Autodesk Inventor part; units mm, degrees
ref_plane "Integral_Raised_Device_Mounting_Boss_StartPlane" through (0, 0, 4) normal (0, 0, 1) x (1, 0, 0)
ref_plane "Device_Clamp_Face_PositiveX" through (33.2942, 0, 0) normal (1, 0, 0) x (0, 1, 0)
ref_plane "Device_Clamp_Face_NegativeX" through (19.7942, 0, 0) normal (1, 0, 0) x (0, 1, 0)
sketch "Continuous_Solid_Plate_No_Openings_Profile" plane through (0, 0, 0) normal (0, 0, 1) x (1, 0, 0)
  line L0 (0, 0) -> (51, 0)
  line L1 (51, 0) -> (51, 80)
  line L2 (51, 80) -> (0, 80)
  line L3 (0, 80) -> (0, 0)
  dimension "d0" = 51
  dimension "d1" = 80
extrude "Continuous_Solid_Plate_No_Openings" add sketch "Continuous_Solid_Plate_No_Openings_Profile" along normal blind 4
ref_plane "Integral_Raised_Device_Mounting_Boss_StartPlane" through (0, 0, 4) normal (0, 0, 1) x (1, 0, 0)
sketch "Integral_Raised_Device_Mounting_Boss_Profile" plane through (0, 0, 4) normal (0, 0, 1) x (1, 0, 0)
  line L0 (19.7942, 4) -> (33.2942, 4)
  line L1 (33.2942, 4) -> (33.2942, 76)
  line L2 (33.2942, 76) -> (19.7942, 76)
  line L3 (19.7942, 76) -> (19.7942, 4)
  point P0 (0, 0)
  dimension "d5" = 19.7943
  dimension "d6" = 4
  dimension "d7" = 13.5
  dimension "d8" = 72
extrude "Integral_Raised_Device_Mounting_Boss" add sketch "Integral_Raised_Device_Mounting_Boss_Profile" along normal blind 6
sketch "Rod_M3_Clearance_8x_Locations" plane through (0, 0, 0) normal (0, 0, 1) x (1, 0, 0)
  circle A0 centre (3, 5) radius 1.7
  circle A1 centre (3, 25) radius 1.7
  circle A2 centre (3, 45) radius 1.7
  circle A3 centre (3, 65) radius 1.7
  circle A4 centre (48, 5) radius 1.7
  circle A5 centre (48, 25) radius 1.7
  circle A6 centre (48, 45) radius 1.7
  circle A7 centre (48, 65) radius 1.7
  point P0 (0, 0)
  dimension "d11" = 3
  dimension "d12" = 5
  dimension "d13" = 3.4
  dimension "d14" = 3
  dimension "d15" = 25
  dimension "d16" = 3.4
  dimension "d17" = 3
  dimension "d18" = 45
  dimension "d19" = 3.4
  dimension "d20" = 3
  dimension "d21" = 65
  dimension "d22" = 3.4
  dimension "d23" = 48
  dimension "d24" = 5
  dimension "d25" = 3.4
  dimension "d26" = 48
  dimension "d27" = 25
  dimension "d28" = 3.4
  dimension "d29" = 48
  dimension "d30" = 45
  dimension "d31" = 3.4
  dimension "d32" = 48
  dimension "d33" = 65
  dimension "d34" = 3.4
extrude "Rod_M3_Clearance_8x" cut sketch "Rod_M3_Clearance_8x_Locations" along normal through all
ref_plane "Device_Clamp_Face_PositiveX" through (33.2942, 0, 0) normal (1, 0, 0) x (0, 1, 0)
sketch "M3_Side_Tap_Locations_PositiveX" plane through (33.2942, 0, 0) normal (1, 0, 0) x (0, 1, 0)
  circle A0 centre (9.828, 7) radius 1.25
  circle A1 centre (25.828, 7) radius 1.25
  circle A2 centre (41.828, 7) radius 1.25
  circle A3 centre (57.828, 7) radius 1.25
  circle A4 centre (73.828, 7) radius 1.25
  point P0 (0, 0)
  dimension "d38" = 9.828
  dimension "d39" = 7
  dimension "d40" = 2.5
  dimension "d41" = 25.828
  dimension "d42" = 7
  dimension "d43" = 2.5
  dimension "d44" = 41.828
  dimension "d45" = 7
  dimension "d46" = 2.5
  dimension "d47" = 57.828
  dimension "d48" = 7
  dimension "d49" = 2.5
  dimension "d50" = 73.828
  dimension "d51" = 7
  dimension "d52" = 2.5
extrude "Device_Tap_Drills_5x_PositiveX" cut sketch "M3_Side_Tap_Locations_PositiveX" against normal blind 6
thread "Device_M3x0_5_6H_PositiveX_1"
thread "Device_M3x0_5_6H_PositiveX_2"
thread "Device_M3x0_5_6H_PositiveX_3"
thread "Device_M3x0_5_6H_PositiveX_4"
thread "Device_M3x0_5_6H_PositiveX_5"
ref_plane "Device_Clamp_Face_NegativeX" through (19.7942, 0, 0) normal (1, 0, 0) x (0, 1, 0)
sketch "M3_Side_Tap_Locations_NegativeX" plane through (19.7942, 0, 0) normal (1, 0, 0) x (0, 1, 0)
  circle A0 centre (9.828, 7) radius 1.25
  circle A1 centre (25.828, 7) radius 1.25
  circle A2 centre (41.828, 7) radius 1.25
  circle A3 centre (57.828, 7) radius 1.25
  circle A4 centre (73.828, 7) radius 1.25
  point P0 (0, 0)
  dimension "d66" = 9.828
  dimension "d67" = 7
  dimension "d68" = 2.5
  dimension "d69" = 25.828
  dimension "d70" = 7
  dimension "d71" = 2.5
  dimension "d72" = 41.828
  dimension "d73" = 7
  dimension "d74" = 2.5
  dimension "d75" = 57.828
  dimension "d76" = 7
  dimension "d77" = 2.5
  dimension "d78" = 73.828
  dimension "d79" = 7
  dimension "d80" = 2.5
extrude "Device_Tap_Drills_5x_NegativeX" cut sketch "M3_Side_Tap_Locations_NegativeX" along normal blind 6
thread "Device_M3x0_5_6H_NegativeX_1"
thread "Device_M3x0_5_6H_NegativeX_2"
thread "Device_M3x0_5_6H_NegativeX_3"
thread "Device_M3x0_5_6H_NegativeX_4"
thread "Device_M3x0_5_6H_NegativeX_5"
equation "\"d0\" = OverallWidth"
equation "\"d1\" = ContactLength"
equation "\"d2\" = BaseThickness"
equation "\"d7\" = FingerWidth"
equation "\"d8\" = ContactLength - 2 * FingerEndInset"
equation "\"d9\" = FingerThickness"
equation "\"d13\" = RodClearanceDiameter"
equation "\"d16\" = RodClearanceDiameter"
equation "\"d19\" = RodClearanceDiameter"
equation "\"d22\" = RodClearanceDiameter"
equation "\"d25\" = RodClearanceDiameter"
equation "\"d28\" = RodClearanceDiameter"
equation "\"d31\" = RodClearanceDiameter"
equation "\"d34\" = RodClearanceDiameter"
equation "\"d40\" = TapDrillDiameter"
equation "\"d43\" = TapDrillDiameter"
equation "\"d46\" = TapDrillDiameter"
equation "\"d49\" = TapDrillDiameter"
equation "\"d52\" = TapDrillDiameter"
equation "\"d53\" = TapDepth"
equation "\"d55\" = TapDepth"
equation "\"d57\" = TapDepth"
equation "\"d59\" = TapDepth"
equation "\"d61\" = TapDepth"
equation "\"d63\" = TapDepth"
equation "\"d68\" = TapDrillDiameter"
equation "\"d71\" = TapDrillDiameter"
equation "\"d74\" = TapDrillDiameter"
equation "\"d77\" = TapDrillDiameter"
equation "\"d80\" = TapDrillDiameter"
equation "\"d81\" = TapDepth"
equation "\"d83\" = TapDepth"
equation "\"d85\" = TapDepth"
equation "\"d87\" = TapDepth"
equation "\"d89\" = TapDepth"
equation "\"d91\" = TapDepth"
equation "\"OverallWidth\" = 51"
equation "\"RodWidth\" = 6"
equation "\"ContactLength\" = 80"
equation "\"BaseThickness\" = 4"
equation "\"FingerStartX\" = 19.79425"
equation "\"FingerWidth\" = 13.5"
equation "\"FingerThickness\" = 6"
equation "\"FingerEndInset\" = 4"
equation "\"RodClearanceDiameter\" = 3.4"
equation "\"ClampFirstY\" = 41.82802"
equation "\"ClampPitch\" = 16"
equation "\"ClampHeight\" = 7"
equation "\"TapDrillDiameter\" = 2.5"
equation "\"TapDepth\" = 6"
equation "\"RodHoleStart\" = 5"
equation "\"RodScrewPitch\" = 20"
equation "\"d4\" = BaseThickness"
equation "\"d37\" = FingerStartX + FingerWidth"
equation "\"d65\" = FingerStartX"
properties part number "Rod_Holder_Adapter"
Check sheet for the modelled part. Datum: model origin and axes. Units: mm. A direction names the side the tool comes from. Round coordinates to 2 decimals unless told otherwise and drop trailing zeros. Order: outer loops, then holes, each group sorted by start corner. A loop starts at its lowest first (then second) coordinate and runs counter-clockwise, first axis right, second up. Notation, with made-up numbers: (-0.5, -14.75) - (27.5, -14.75) arc R31 ccw to (27.5, 19.25) - close; hole circle Ø8 at (70.5, 18). An arc over 180 degrees is marked (long way). Answer as CSV lines item,"result". Start each with the question number.
1) Tool access check on faces 1 (the face through (25.794, 10, 7)), 2 (the face through (51, 39, 2)), 3 (the face through (27.294, 10, 7)). Record the directions out of +Z, -Z, +X, -X, +Y, -Y that give a thin tool (end or side, any length) a straight path to the whole face; none if there is none.
2) Section check D-D (x = 3). Record the cut outline in (y, z), then the cut area to 3 significant figures.
3) Scan lines: probe 1 along Y at (x, z) = (3, 3); probe 2 along X at (y, z) = (45, 2.6); probe 3 along Z at (x, y) = (9, 7). Record each from-to range of solid material in increasing order.
4) Draft check along Z on faces 4 (the face through (22.752, 74.983, 7.479)), 5 (the face through (22.752, 8.836, 7.761)), 6 (the face through (46.75, 63.85, 1.97)). Enter one of: +Z half, -Z half, draft (parallel to the pull), parting line (faces both ways), or undercut.
5) Section check A-A (y = 45). Record the cut outline in (x, z), then the cut area to 3 significant figures.
6) Depth check by flat-ended pin: pin 1 (1.5 mm diameter, centred on y = 57.828, z = 7, fed in from +X); pin 2 (4 mm diameter, centred on x = 48, y = 65, fed in from +Z); pin 3 (4 mm diameter, centred on x = 18, y = 20, fed in from -Z); pin 4 (5 mm diameter, centred on y = 37, z = 8, fed in from +X). Enter the tip coordinate at first touch or a pass-through.
7) Section check B-B (x = 30.5). Record the cut outline in (y, z), then the cut area to 3 significant figures.
8) Section check C-C (z = 2.25). Give the number of separate pieces and of enclosed holes in the cut face, then the cut area to 3 significant figures.
Determined:
1,face 1,"-X"
1,face 2,"+Z, -Z, +X, +Y, -Y"
1,face 3,"+X"
2,outline,"(0, 0) - (3.3, 0) - (3.3, 4) - (0, 4) - close; (6.7, 0) - (23.3, 0) - (23.3, 4) - (6.7, 4) - close; (26.7, 0) - (43.3, 0) - (43.3, 4) - (26.7, 4) - close; (46.7, 0) - (63.3, 0) - (63.3, 4) - (46.7, 4) - close; (66.7, 0) - (80, 0) - (80, 4) - (66.7, 4) - close"
2,area,"266 mm^2"
3,probe 1,"0 to 3.3, 6.7 to 23.3, 26.7 to 43.3, 46.7 to 63.3, 66.7 to 80"
3,probe 2,"0 to 1.3, 4.7 to 46.3, 49.7 to 51"
3,probe 3,"0 to 4"
4,face 4,"undercut"
4,face 5,"undercut"
4,face 6,"draft"
5,outline,"(0, 0) - (1.3, 0) - (1.3, 4) - (0, 4) - close; (4.7, 0) - (46.3, 0) - (46.3, 4) - (33.29, 4) - (33.29, 10) - (19.79, 10) - (19.79, 4) - (4.7, 4) - close; (49.7, 0) - (51, 0) - (51, 4) - (49.7, 4) - close"
5,area,"258 mm^2"
6,pin 1,"x = 27.29"
6,pin 2,"z = 4"
6,pin 3,"z = 0"
6,pin 4,"x = 33.29"
7,outline,"(0, 0) - (80, 0) - (80, 4) - (76, 4) - (76, 10) - (4, 10) - (4, 4) - (0, 4) - close; hole circle Ø2.5 at (9.83, 7); hole circle Ø2.5 at (25.83, 7); hole circle Ø2.5 at (41.83, 7); hole circle Ø2.5 at (57.83, 7); hole circle Ø2.5 at (73.83, 7)"
7,area,"727 mm^2"
8,separate pieces,"1"
8,enclosed holes,"8"
8,area,"4,010 mm^2"
